Autodesk Inventor part; units mm, degrees
ref_plane "1_XY" through (27.0002, 0, 0) normal (1, 0, 0) x (0, 0, -1)
ref_plane "1_YZ" through (27.0002, 0, 0) normal (0, 0, -1) x (0, 1, 0)
ref_plane "1_ZX" through (27.0002, 0, 0) normal (0, 1, 0) x (1, 0, 0)
sketch "Sketch_8" plane through (0, 0, 0) normal (0, 0, 1) x (1, 0, 0)
  line L0 (24.6126, 0) -> (0, 0)
  line L1 (0, 0) -> (0, 8.9091)
  line L2 (0, 8.9091) -> (0.762, 9.671)
  line L3 (0.762, 9.671) -> (4.0386, 9.671)
  line L4 (4.0386, 9.671) -> (4.8006, 8.9091)
  line L5 (4.8006, 8.9091) -> (5.5626, 8.9091)
  line L6 (5.5626, 8.9091) -> (5.5626, 10.3759)
  line L7 (5.5626, 10.3759) -> (8.7363, 10.3759)
  line L8 (8.7363, 10.3759) -> (9.3142, 10.9537)
  line L9 (9.3142, 10.9537) -> (23.8506, 10.9537)
  line L10 (23.8506, 10.9537) -> (24.6126, 10.1918)
  line L11 (24.6126, 10.1918) -> (24.6126, 0)
  line L12 (24.6126, 0) -> (0, 0)
revolve "Revolution1" add sketch "Sketch_8" angle 360 about axis through (24.6126, 0, 0) along (1, 0, 0)
sketch "Sketch_15" plane through (0, 0, 0) normal (0, 0, 1) x (1, 0, 0)
  line L0 (40.4876, 0) -> (24.6126, 0)
  line L1 (24.6126, 0) -> (24.6126, 7.9057)
  line L2 (24.6126, 7.9057) -> (27.0002, 7.9057)
  line L3 (27.0002, 7.9057) -> (27.0002, 7.7279)
  arc A0 (27.0002, 7.7279) -> (27.8892, 6.839) centre (27.8892, 7.7279) ccw
  line L4 (27.8892, 6.839) -> (29.1719, 6.839)
  arc A1 (29.1719, 6.839) -> (29.7706, 7.0708) centre (29.1719, 7.7279) ccw
  line L5 (29.7706, 7.0708) -> (29.8005, 7.098)
  line L6 (29.8005, 7.098) -> (30.64, 7.9375)
  line L7 (30.64, 7.9375) -> (39.6481, 7.9375)
  line L8 (39.6481, 7.9375) -> (40.4876, 7.098)
  line L9 (40.4876, 7.098) -> (40.4876, 0)
  line L10 (40.4876, 0) -> (24.6126, 0)
revolve "Revolution2" add sketch "Sketch_15" angle 360 about axis through (40.4876, 0, 0) along (1, 0, 0)
thread "Thread1"
sketch "Sketch_9" plane through (40.4876, 0, 0) normal (1, 0, 0) x (0, 0, -1)
  line L0 (-21.9075, -43.815) -> (21.9075, -43.815)
  line L1 (21.9075, -43.815) -> (21.9075, 43.815)
  line L2 (21.9075, 43.815) -> (-21.9075, 43.815)
  line L3 (-21.9075, 43.815) -> (-21.9075, -43.815)
  line L4 (-4.7307, -21.9075) -> (4.7307, -21.9075)
  line L5 (4.7307, -21.9075) -> (4.7307, 21.9075)
  line L6 (4.7307, 21.9075) -> (-4.7307, 21.9075)
  line L7 (-4.7307, 21.9075) -> (-4.7307, -21.9075)
extrude "Extrusion1" cut sketch "Sketch_9" against normal blind 15.875
sketch "Sketch4" plane through (0, 0, 0) normal (-1, 0, 0) x (0, 0, 1)
  point P0 (0, 0)
hole "Hole1" at (0, 0, 0) direction (1, 0, 0) diameter 7.9248 depth 23.5814 tip angle 120
sketch "Sketch_47" plane through (0, 0, 0) normal (0, 0, 1) x (1, 0, 0)
  line L0 (17.4752, 0) -> (17.4752, 10.9537)
  line L1 (17.4752, 10.9537) -> (22.9299, 10.9537)
  line L2 (22.9299, 10.9537) -> (22.2949, 10.3187)
  line L3 (22.2949, 10.3187) -> (22.04, 2.1565)
  line L4 (22.04, 2.1565) -> (22.04, 0)
  line L5 (22.04, 0) -> (17.4752, 0)
  line L6 (17.4752, 0) -> (17.4752, 10.9537)
revolve "Revolution3" cut sketch "Sketch_47" angle 360 about axis through (17.4752, 0, 0) along (0, -1, 0)
thread "Thread2"
sketch "Sketch_24" plane through (0, 0, 0) normal (0, 0, 1) x (1, 0, 0)
  line L0 (5.5626, 0) -> (4.8006, 0)
  line L1 (4.4955, 10.3759) -> (4.4955, 10.2917)
  line L2 (4.4955, 10.2917) -> (5.4401, 9.3472)
  arc A0 (5.4401, 9.1676) -> (5.4401, 9.3472) centre (5.3503, 9.2574) ccw
  line L3 (5.4401, 9.1676) -> (5.1816, 8.9091)
  line L4 (5.1816, 8.9091) -> (4.8006, 8.9091)
  line L5 (4.8006, 8.9091) -> (4.8006, 8.655)
  line L6 (4.8006, 8.655) -> (5.5626, 8.655)
  line L7 (5.5626, 8.655) -> (5.5626, 9.512)
  line L8 (5.5626, 9.512) -> (4.6987, 10.3759)
  line L9 (4.6987, 10.3759) -> (4.4955, 10.3759)
revolve "Revolution4" add sketch "Sketch_24" angle 360 about axis through (5.5626, 0, 0) along (1, 0, 0)
sketch "Sketch_43" plane through (0, 0, 0) normal (0, 0, 1) x (1, 0, 0)
  circle A0 centre (33.3248, 0) radius 3.2004
extrude "Extrusion2" cut sketch "Sketch_43" along normal mid plane 14.1922
ref_plane "1_XY" through (27.0002, 0, 0) normal (1, 0, 0) x (0, 0, -1)
ref_plane "1_YZ" through (27.0002, 0, 0) normal (0, 0, -1) x (0, 1, 0)
ref_plane "1_ZX" through (27.0002, 0, 0) normal (0, 1, 0) x (1, 0, 0)
ref_plane "c1_XY" through (24.6126, 7.9057, 0) normal (0, 0, 1) x (1, 0, 0)
ref_plane "c1_YZ" through (24.6126, 7.9057, 0) normal (1, 0, 0) x (0, 1, 0)
ref_plane "c1_ZX" through (24.6126, 7.9057, 0) normal (0, 1, 0) x (0, 0, 1)
ref_plane "c2_XY" through (24.6126, -7.9057, 0) normal (0, 0, 1) x (1, 0, 0)
ref_plane "c2_YZ" through (24.6126, -7.9057, 0) normal (1, 0, 0) x (0, 1, 0)
ref_plane "c2_ZX" through (24.6126, -7.9057, 0) normal (0, 1, 0) x (0, 0, 1)
ref_plane "cc1_XY" through (24.6126, 0, 0) normal (0, 0, 1) x (1, 0, 0)
ref_plane "cc1_YZ" through (24.6126, 0, 0) normal (1, 0, 0) x (0, 1, 0)
ref_plane "cc1_ZX" through (24.6126, 0, 0) normal (0, 1, 0) x (0, 0, 1)
ref_plane "cc2_XY" through (27.0002, 0, 0) normal (0, 0, 1) x (1, 0, 0)
ref_plane "cc2_YZ" through (27.0002, 0, 0) normal (1, 0, 0) x (0, 1, 0)
ref_plane "cc2_ZX" through (27.0002, 0, 0) normal (0, 1, 0) x (0, 0, 1)
ref_plane "lovra1_XY" through (35.7124, 0, 0) normal (1, 0, 0) x (0, 0, -1)
ref_plane "lovra1_YZ" through (35.7124, 0, 0) normal (0, 0, -1) x (0, 1, 0)
ref_plane "lovra1_ZX" through (35.7124, 0, 0) normal (0, 1, 0) x (1, 0, 0)
ref_plane "lovra2_XY" through (35.7124, 7.874, 0) normal (1, 0, 0) x (0, 0, -1)
ref_plane "lovra2_YZ" through (35.7124, 7.874, 0) normal (0, 0, -1) x (0, 1, 0)
ref_plane "lovra2_ZX" through (35.7124, 7.874, 0) normal (0, 1, 0) x (1, 0, 0)
ref_plane "lovra21_XY" through (0, 0, 5.2705) normal (1, 0, 0) x (0, 0, -1)
ref_plane "lovra21_YZ" through (0, 0, 5.2705) normal (0, 0, -1) x (0, 1, 0)
ref_plane "lovra21_ZX" through (0, 0, 5.2705) normal (0, 1, 0) x (1, 0, 0)
ref_plane "lovra22_XY" through (0, 0, -5.2705) normal (1, 0, 0) x (0, 0, -1)
ref_plane "lovra22_YZ" through (0, 0, -5.2705) normal (0, 0, -1) x (0, 1, 0)
ref_plane "lovra22_ZX" through (0, 0, -5.2705) normal (0, 1, 0) x (1, 0, 0)
ref_plane "lovra3_XY" through (35.7124, -7.874, 0) normal (1, 0, 0) x (0, 0, -1)
ref_plane "lovra3_YZ" through (35.7124, -7.874, 0) normal (0, 0, -1) x (0, 1, 0)
ref_plane "lovra3_ZX" through (35.7124, -7.874, 0) normal (0, 1, 0) x (1, 0, 0)
ref_plane "olen_XY" through (33.3248, 0, 0) normal (1, 0, 0) x (0, 0, -1)
ref_plane "olen_YZ" through (33.3248, 0, 0) normal (0, 0, -1) x (0, 1, 0)
ref_plane "olen_ZX" through (33.3248, 0, 0) normal (0, 1, 0) x (1, 0, 0)
ref_plane "p1_XY" through (40.4876, 0, 4.7307) normal (1, 0, 0) x (0, 0, -1)
ref_plane "p1_YZ" through (40.4876, 0, 4.7307) normal (0, 0, -1) x (0, 1, 0)
ref_plane "p1_ZX" through (40.4876, 0, 4.7307) normal (0, 1, 0) x (1, 0, 0)
ref_plane "p2_XY" through (40.4876, 0, -4.7307) normal (1, 0, 0) x (0, 0, -1)
ref_plane "p2_YZ" through (40.4876, 0, -4.7307) normal (0, 0, -1) x (0, 1, 0)
ref_plane "p2_ZX" through (40.4876, 0, -4.7307) normal (0, 1, 0) x (1, 0, 0)
ref_plane "port_XY" through (17.4752, 10.9537, 0) normal (0, 0, 1) x (1, 0, 0)
ref_plane "port_YZ" through (17.4752, 10.9537, 0) normal (1, 0, 0) x (0, 1, 0)
ref_plane "port_ZX" through (17.4752, 10.9537, 0) normal (0, 1, 0) x (0, 0, 1)
ref_plane "port2_XY" through (40.4876, 0, 0) normal (1, 0, 0) x (0, 0, -1)
ref_plane "port2_YZ" through (40.4876, 0, 0) normal (0, 0, -1) x (0, 1, 0)
ref_plane "port2_ZX" through (40.4876, 0, 0) normal (0, 1, 0) x (1, 0, 0)
ref_plane "thd1_XY" through (40.4876, 0, 7.9375) normal (1, 0, 0) x (0, 0, -1)
ref_plane "thd1_YZ" through (40.4876, 0, 7.9375) normal (0, 0, -1) x (0, 1, 0)
ref_plane "thd1_ZX" through (40.4876, 0, 7.9375) normal (0, 1, 0) x (1, 0, 0)
ref_plane "thd2_XY" through (40.4876, 0, -7.9375) normal (1, 0, 0) x (0, 0, -1)
ref_plane "thd2_YZ" through (40.4876, 0, -7.9375) normal (0, 0, -1) x (0, 1, 0)
ref_plane "thd2_ZX" through (40.4876, 0, -7.9375) normal (0, 1, 0) x (1, 0, 0)
ref_plane "to_mounting_bracket_XY" through (24.6126, 0, 0) normal (1, 0, 0) x (0, 0, -1)
ref_plane "to_mounting_bracket_YZ" through (24.6126, 0, 0) normal (0, 0, -1) x (0, 1, 0)
ref_plane "to_mounting_bracket_ZX" through (24.6126, 0, 0) normal (0, 1, 0) x (1, 0, 0)
ref_plane "to_nut_XY" through (27.0002, 0, 0) normal (1, 0, 0) x (0, 0, -1)
ref_plane "to_nut_YZ" through (27.0002, 0, 0) normal (0, 0, -1) x (0, 1, 0)
ref_plane "to_nut_ZX" through (27.0002, 0, 0) normal (0, 1, 0) x (1, 0, 0)
ref_plane "to_pin_XY" through (33.3248, 0, 0) normal (0, 0, 1) x (1, 0, 0)
ref_plane "to_pin_YZ" through (33.3248, 0, 0) normal (1, 0, 0) x (0, 1, 0)
ref_plane "to_pin_ZX" through (33.3248, 0, 0) normal (0, 1, 0) x (0, 0, 1)
ref_plane "to_screw_XY" through (17.4752, -6.0452, -2.032) normal (0, 0, -1) x (1, 0, 0)
ref_plane "to_screw_YZ" through (17.4752, -6.0452, -2.032) normal (1, 0, 0) x (0, -1, 0)
ref_plane "to_screw_ZX" through (17.4752, -6.0452, -2.032) normal (0, -1, 0) x (0, 0, -1)
ref_plane "to_tube_XY" through (4.8006, 0, 0) normal (1, 0, 0) x (0, 0, -1)
ref_plane "to_tube_YZ" through (4.8006, 0, 0) normal (0, 0, -1) x (0, 1, 0)
ref_plane "to_tube_ZX" through (4.8006, 0, 0) normal (0, 1, 0) x (1, 0, 0)
properties part number "04P0K000_rear_head"
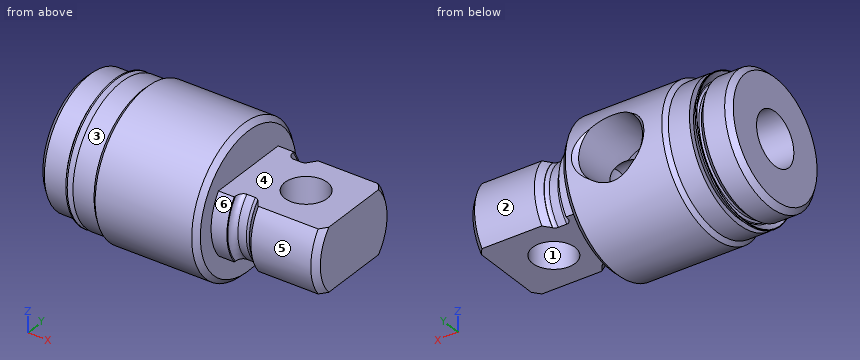
Source: CAD feature listing. Evaluate the final solid. Frame: model axes, mm. Face numbers are marked on the shaded views. A direction names the side the tool comes from. Give positions to 0.01 mm unless a question says otherwise; leave off trailing zeros. Order: outer loops, then holes, each group sorted by start corner. A loop starts at its lowest first (then second) coordinate and runs counter-clockwise, first axis right, second up. Notation, with made-up numbers: (79, 32.25) -> (114, 32.25) arc R17 cw to (114, 47.25) -> close; hole circle Ø7 at (-31.5, 62.25). An arc over 180 degrees is marked (long way). Use a Markdown table: item, result.
Q1. Access query for the marked faces 4, 5 and 6. Directions: +Z, -Z, +X, -X, +Y, -Y. A direction counts if a zero-diameter tool reaches every point of the face in a straight line with its end or side. Return the directions, or none.
A:
| item | result |
|---|---|
| face 4 | +Z, +X, +Y, -Y |
| face 5 | +X, -Y |
| face 6 | -Y |
Q2. Pull-direction query (Y, two-part tool) for the marked faces 1, 2 and 3; classes: +Y half, -Y half, draft (parallel to the pull), parting line (faces both ways), or undercut.
A:
| item | result |
|---|---|
| face 1 | undercut |
| face 2 | +Y half |
| face 3 | parting line |
Q3. Section B-B (z = -1). State how many separate pieces and enclosed holes the cut face has, and give its area (3 significant figures).
A:
| item | result |
|---|---|
| separate pieces | 2 |
| enclosed holes | 1 |
| area | 473 mm^2 |
Q4. Section C-C (x = 38.5). Return the cut outline in (y, z) (1 decimal), and give its area (3 significant figures).
A:
| item | result |
|---|---|
| outline | (-6.4, -4.7) -> (6.4, -4.7) arc R7.9 ccw to (6.4, 4.7) -> (-6.4, 4.7) arc R7.9 ccw to start |
| area | 141 mm^2 |
Q5. Material intervals for line 1 (Z direction, x = 12.75, y = 0); line 2 (X direction, y = -7.5, z = 0.5); line 3 (Z direction, x = 19, y = -1.5), sorted ascending. Write a range as [from, to].
A:
| item | result |
|---|---|
| line 1 | [-10.95, -3.96], [3.96, 10.95] |
| line 2 | [0, 27.03], [30.22, 40.07] |
| line 3 | [-10.85, -3.67], [3.67, 10.85] |
Q6. Section A-A (x = 8). Return the cut outline in (y, z), and give its area (3 significant figures).
A:
| item | result |
|---|---|
| outline | circle Ø20.75 at (0, 0); hole circle Ø7.92 at (0, 0) |
| area | 289 mm^2 |
Q7. First-contact query: P1, Ø4, axis at x = 32.5, y = 1.5, coming from the -Z side; P2, Ø2, axis at x = 17.5, z = 8, coming from the +Y side; P3, Ø6.5, axis at x = 32, y = -1.5, coming from the +Z side. Flat tips, straight axial feed; report the tip coordinate or a pass-through.
A:
| item | result |
|---|---|
| P1 | z = -4.73 |
| P2 | y = 8.43 |
| P3 | z = 4.73 |
